Geometry check sheet. Reference: the model listing, model coordinates, mm. Face numbers are marked on the shaded views. A direction names the side the tool comes from. Give positions to 0.01 mm unless a question says otherwise; leave off trailing zeros. Order: outer loops, then holes, each group sorted by start corner. A loop starts at its lowest first (then second) coordinate and runs counter-clockwise, first axis right, second up. Notation, with made-up numbers: M -15.75,-11 L -8.75,-11 A27 cw -8.75,20 Z; hole C 58.25,31.25 d11. An arc over 180 degrees is marked long. Answer as CSV lines item,"result". Start each with the question number.
Q1. Thickness scan on line 1 (Z direction, x = -1.5, y = 6); line 2 (Y direction, x = 2, z = 2.75); line 3 (X direction, y = 6.75, z = 1). Record the ranges inside material, lowest first.
Q2. Section check A-A, the plane x = 0. Record the boundary of the cut face in (y, z), then the cut area to 3 significant figures.
Q3. Section check D-D, the plane y = 11. Record the boundary of the cut face in (x, z).
Q4. Set-up check for the marked faces 1 and 2: record each of +Z, -Z, +X, -X, +Y, -Y from which the full face is reachable in a straight line by a thin tool's end or side.
Q5. Mould release check, pull along X, two halves, no side actions. Record for the marked faces 3, 4 and 5: +X half, -X half, draft (parallel to the pull), parting line (faces both ways), or undercut.
Q6. Section check C-C, the plane y = 3.5. Record the boundary of the cut face in (x, z).
Q7. Section check B-B, the plane z = 0. Record the boundary of the cut face in (x, y), then the cut area to 3 significant figures.
Q8. Go/stop test with flat-tipped pins: pin 1 (4 mm diameter, centred on x = -2.5, y = 5.5, fed in from -Z); pin 2 (1 mm diameter, centred on y = 11.5, z = -1.5, fed in from -X); pin 3 (1 mm diameter, centred on y = 5.5, z = -0.5, fed in from +X); pin 4 (4 mm diameter, centred on x = 0, z = 0, fed in from +Y). Record where each tip stops, or that it passes through.
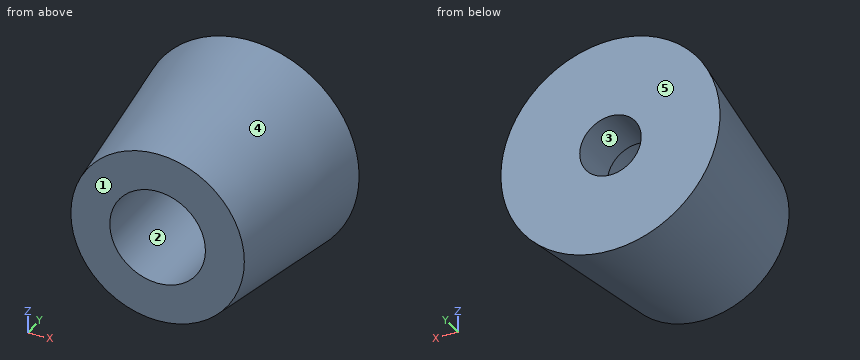
```python
from build123d import *

# Parameters (mm, degrees)
SKETCH1_R           = 6.35
BOSS_EXTRUDE1_DEPTH = 12.7
BOSS_EXTRUDE1_DRAFT = -7.5
SKETCH2_R           = 3.5
CUT_EXTRUDE1_DEPTH  = 8.89
SKETCH3_R           = 2.25
CUT_EXTRUDE2_DEPTH  = 18.029226108


with BuildPart() as part:
    # Sketch1 → Boss-Extrude1 (with draft: the straight prism first)
    with BuildSketch(Plane(origin=(0, 0, 0), x_dir=(1, 0, 0), z_dir=(0, 1, 0))):
        Circle(SKETCH1_R)
    extrude(amount=BOSS_EXTRUDE1_DEPTH)
    # Boss-Extrude1: the draft: its side faces are tilted about the plane it starts from
    boss_extrude1_sides = [part.faces().sort_by_distance(p)[0] for p in [
        (-6.35, 6.35, 0),
    ]]
    draft(boss_extrude1_sides, Plane(origin=(0, 0, 0), x_dir=(1, 0, 0), z_dir=(0, 1, 0)), BOSS_EXTRUDE1_DRAFT)

    # Sketch2 → Cut-Extrude1 (cut)
    with BuildSketch(Plane.XZ):
        with Locations(Location((0, 0, 0), (0, 0, 270))):
            Circle(SKETCH2_R)
    extrude(amount=-CUT_EXTRUDE1_DEPTH, mode=Mode.SUBTRACT)

    # Sketch3 → Cut-Extrude2 (cut, through all)
    with BuildSketch(Plane(origin=(0, 12.7, 0), x_dir=(1, 0, 0), z_dir=(0, 1, 0))):
        with Locations(Location((0, 0, 0), (0, 0, 270))):
            Circle(SKETCH3_R)
    extrude(amount=-CUT_EXTRUDE2_DEPTH, mode=Mode.SUBTRACT)


solid = part.part
```
Answer block:
1,line 1,"z = -6.98 to -3.16, 3.16 to 6.98"
1,line 2,"y = 8.89 to 12.7"
1,line 3,"x = -7.17 to -3.35, 3.35 to 7.17"
2,outline,"M 0,-6.35 L 12.7,-8.02 L 12.7,-2.25 L 8.89,-2.25 L 8.89,-3.5 L 0,-3.5 Z; M 0,3.5 L 8.89,3.5 L 8.89,2.25 L 12.7,2.25 L 12.7,8.02 L 0,6.35 Z"
2,area,"103 mm2"
3,outline,"C 0,0 d15.6; hole C 0,0 d4.5"
4,face 1,"+Z, -Z, +X, -X, -Y"
4,face 2,"-Y"
5,face 3,"undercut"
5,face 4,"parting line"
5,face 5,"draft"
6,outline,"C 0,0 d13.62; hole C 0,0 d7"
7,outline,"M -8.02,12.7 L -6.35,0 L -3.5,0 L -3.5,8.89 L -2.25,8.89 L -2.25,12.7 Z; M 2.25,8.89 L 3.5,8.89 L 3.5,0 L 6.35,0 L 8.02,12.7 L 2.25,12.7 Z"
7,area,"103 mm2"
8,pin 1,"stops at z = -7.18"
8,pin 2,"stops at x = -7.83"
8,pin 3,"stops at x = 7.13"
8,pin 4,"passes through"
